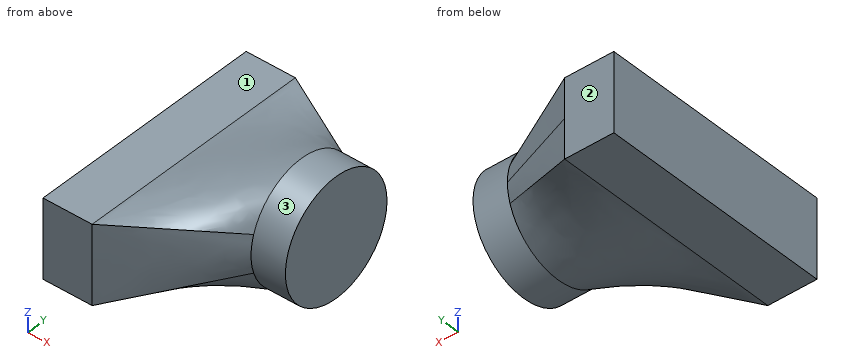
from build123d import *

# Parameters (mm, degrees)
SKETCH003_R  = 76.2
PAD001_DEPTH = 44.45
SKETCH_W     = 304.8
SKETCH_H     = 101.6
SKETCH001_R  = 76.2
SKETCH004_W  = 304.8
SKETCH004_H  = 101.6
PAD_DEPTH    = 63.5


with BuildPart() as part:
    # Sketch003 → Pad001 (new body)
    with BuildSketch(Plane.YZ.offset(254)):
        Circle(SKETCH003_R)
    extrude(amount=PAD001_DEPTH)

    # Sketch → AdditiveLoft section 0
    with BuildSketch(Plane.YZ.offset(114.3)):
        with Locations((0, -38.1)):
            Rectangle(SKETCH_W, SKETCH_H)
    # Sketch001 → AdditiveLoft section 1
    with BuildSketch(Plane.YZ.offset(254)):
        Circle(SKETCH001_R)
    loft()

    # Sketch004 → Pad (join)
    with BuildSketch(Plane.YZ.offset(114.3)):
        with Locations((0, -38.1)):
            Rectangle(SKETCH004_W, SKETCH004_H)
    extrude(amount=-PAD_DEPTH)


solid = part.part
Work out the finished part from the listing and answer in its coordinate system (mm). Face numbers are marked on the shaded views. A direction names the side the tool comes from. Give positions to 0.01 mm unless a question says otherwise; leave off trailing zeros. One line per item, written item: value. Start each with the question number.
1. Consider probe 1 along Z at (x, y) = (77.5, -3.5); probe 2 along Z at (x, y) = (135, 113.5); probe 3 along Y at (x, z) = (134, -20). Determine where each line is inside the solid, lowest interval first.
2. For the marked faces 1, 2 and 3, determine the directions among +Z, -Z, +X, -X, +Y, -Y from which every point of the face is accessible in a straight line to the end or side of a thin tool.
3. Given pin 1 (4 mm diameter, centred on x = 136.5, z = 11.5, fed in from -Y); pin 2 (6 mm diameter, centred on x = 164, z = 6.5, fed in from -Y); pin 3 (3 mm diameter, centred on x = 136.5, z = -61.5, fed in from +Y), each flat-ended and moving along its own axis, determine where each tip first touches the part or whether it passes through.
Geometry results:
1. probe 1: -88.9 to 12.7
1. probe 2: -81.82 to 16.91
1. probe 3: -141.61 to 141.61
2. face 1: +Z, -X, +Y, -Y
2. face 2: +Z, -Z, +X, -X, +Y
2. face 3: +X
3. pin 1: y = -140.88
3. pin 2: y = -126.18
3. pin 3: y = 140.89
